Autodesk Inventor part; units mm, degrees
ref_plane "YZ Plane" through (0, 0, 0) normal (1, 0, 0) x (0, 1, 0)
ref_plane "XZ Plane" through (0, 0, 0) normal (0, 1, 0) x (-1, 0, 0)
ref_plane "XY Plane" through (0, 0, 0) normal (0, 0, 1) x (1, 0, 0)
sketch "Sketch1" plane through (0, 0, 0) normal (1, 0, 0) x (0, 1, 0)
  circle A0 centre (15, 10) radius 1.65
  line L0 (0, 0) -> (9.4364, 0)
  circle A1 centre (15, -10) radius 1.65
  line L1 (0, 20) -> (23, 20)
  line L2 (23, 20) -> (23, -20)
  line L3 (23, -20) -> (0, -20)
  line L4 (0, -20) -> (0, 20)
  dimension "d0" = 15
  dimension "d1" = 20
  dimension "d2" = 3.3
  dimension "d3" = 23
  dimension "d4" = 40
extrude "Extrusion1" add sketch "Sketch1" along normal blind 6
sketch "Sketch2" plane through (6, 0, 0) normal (1, 0, 0) x (0, 0, -1)
  line L0 (20, 23) -> (-20, 23)
  line L1 (-20, 23) -> (-20, 0)
  line L2 (-20, 0) -> (20, 0)
  line L3 (20, 0) -> (20, 23)
  circle A0 centre (-10, 15) radius 1.65
  circle A1 centre (10, 15) radius 1.65
  line L4 (-20, 0) -> (20, 0)
  line L5 (20, 0) -> (20, 6)
  line L6 (20, 6) -> (-20, 6)
  line L7 (-20, 6) -> (-20, 0)
  point P0 (0, 0)
  dimension "d7" = 6
extrude "Extrusion2" add sketch "Sketch2" along normal blind 20 contours L3 L2 L1 L6
sketch "Sketch3" plane through (6, 6, 20) normal (0, 1, 0) x (1, 0, 0)
  line L0 (0, 0) -> (0, 40)
  line L1 (0, 0) -> (20, 0)
  line L2 (20, 40) -> (20, 0)
  line L3 (0, 40) -> (20, 40)
  circle A0 centre (10, 13.35) radius 1.65
  circle A1 centre (10, 26.65) radius 1.65
  line L4 (10, 13.35) -> (10, 26.65) construction
  point P0 (-6, 20)
  point P1 (10, 40)
  point P2 (10, 20)
  point P3 (0, 20)
  dimension "d10" = 3.3
  dimension "d11" = 10
extrude "Extrusion3" cut sketch "Sketch3" against normal through all contours A0 | A1
chamfer "Chamfer1" distance 2 angle 45 5 edges at (3, 23, 20) (3, 23, -20) (26, 3, 20) (26, 3, -20) (6, 6, 0)
properties part number "SOPORTE_TOBOGAN_V2" material "Steel, Mild, Welded"
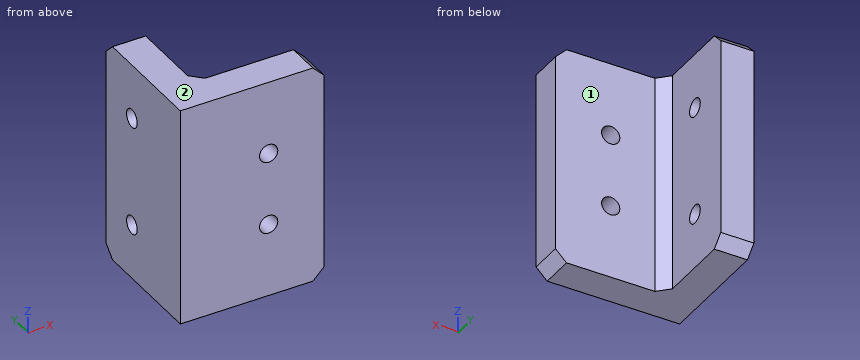
Could you check a few things on this model? Use its own coordinates, in mm. Face numbers are marked on the shaded views. A direction names the side the tool comes from. Give positions to 0.01 mm unless a question says otherwise; leave off trailing zeros. Loops run counter-clockwise (first coordinate to the right, second up) from the corner with the lowest first, then second, coordinate; pieces in that order, holes last. Notation, with made-up numbers: (30.5, 78.25) -> (50.5, 78.25) arc R31 cw to (50.5, 106.25) -> close; hole circle Ø7 at (5, -17). An arc over 180 degrees is marked (long way). Return JSON: item names as keys, results as strings.
Item 1: Which directions (+Z, -Z, +X, -X, +Y, -Y) give clear straight access to the entire face, cutting with the end or side of a thin tool? Please do the marked faces 1 and 2.
Geometry results:
{"face 1": "+Z, -Z, +X, +Y", "face 2": "+Z, +X, -X, +Y, -Y"}
Item 2: I'm going to push flat-ended pins straight in: pin 1 (6 mm diameter, centred on y = 16, z = 10.5, fed in from +X); pin 2 (5.5 mm diameter, centred on x = 18, z = -0.5, fed in from +Y); pin 3 (2 mm diameter, centred on x = 16, z = 6.65, fed in from -Y). Where does each tip first touch, or does it pass through?
Geometry results:
{"pin 1": "stops at x = 6", "pin 2": "stops at y = 6", "pin 3": "passes through"}
Item 3: If we section it at D-D on x = 16: List the corners of the cut face in (y, z) for me, plus the area to 3 significant figures.
Geometry results:
{"outline": "(0, -20) -> (6, -20) -> (6, -8.3) -> (0, -8.3) -> close; (0, -5) -> (6, -5) -> (6, 5) -> (0, 5) -> close; (0, 8.3) -> (6, 8.3) -> (6, 20) -> (0, 20) -> close", "area": "200 mm²"}
Item 4: If we section it at B-B on z = 10: List the corners of the cut face in (x, y) for me, plus the area to 3 significant figures.
Geometry results:
{"outline": "(0, 0) -> (26, 0) -> (26, 6) -> (8, 6) -> (6, 8) -> (6, 13.35) -> (0, 13.35) -> close; (0, 16.65) -> (6, 16.65) -> (6, 23) -> (0, 23) -> close", "area": "240 mm²"}
Item 5: If we section it at A-A on x = 4.25: List the corners of the cut face in (y, z) for me.
Geometry results:
{"outline": "(0, -20) -> (21, -20) -> (23, -18) -> (23, 18) -> (21, 20) -> (0, 20) -> close; hole circle Ø3.3 at (15, -10); hole circle Ø3.3 at (15, 10)"}
Item 6: If we section it at C-C on y = 15: List the corners of the cut face in (x, z) for me.
Geometry results:
{"outline": "(0, -20) -> (6, -20) -> (6, -11.65) -> (0, -11.65) -> close; (0, -8.35) -> (6, -8.35) -> (6, 8.35) -> (0, 8.35) -> close; (0, 11.65) -> (6, 11.65) -> (6, 20) -> (0, 20) -> close"}
Item 7: I need wall thicknesses on L1, parallel to Z at x = 16, y = 1.55; L2, parallel to Z at x = 4.35, y = 15; L3, parallel to X at y = 1.5, z = 6.65. Which ranges of each line are inside material? Lowest first, please. Write a range as from..to.
Geometry results:
{"L1": "z = -20..-8.3, -5..5, 8.3..20", "L2": "z = -20..-11.65, -8.35..8.35, 11.65..20", "L3": "x = 0..14.35, 17.65..26"}
